For this review, take the finished solid that the model builds, in its own axes (mm). A direction names the side the tool comes from. Round coordinates to 2 decimals unless told otherwise and drop trailing zeros. Order: outer loops, then holes, each group sorted by start corner. A loop starts at its lowest first (then second) coordinate and runs counter-clockwise, first axis right, second up. Notation, with made-up numbers: (73.5, 36.5) - (85.5, 36.5) arc R21 ccw to (85.5, 74.5) - close; hole circle Ø4 at (-28.75, 1.5). An arc over 180 degrees is marked (long way). One line per item, written item: value.
```python
from build123d import *

# Parameters (mm, degrees)
BOSS_EXTRU_1_DEPTH = 20
ESQUISSE2_R        = 3
BOSS_EXTRU_2_DEPTH = 5


with BuildPart() as part:
    # Esquisse1 → Boss.-Extru.1 (new body)
    with BuildSketch(Plane(origin=(0, 0, 0), x_dir=(1, 0, 0), z_dir=(0, 1, 0))):
        Polygon((0, 0), (40, 0), (40, 2), (47, 2), (47, 7), (40, 7), (40, 28), (47, 28), (47, 31.5), (40, 31.5), (40, 37), (0, 37), (0, 31.5), (-7, 31.5), (-7, 28), (0, 28), align=None)
    extrude(amount=BOSS_EXTRU_1_DEPTH)

    # Esquisse2 → Boss.-Extru.2 (add)
    with BuildSketch(Plane(origin=(0, 0, -37), x_dir=(-1, 0, 0), z_dir=(0, 0, -1))):
        with Locations((-30, 10)):
            Circle(ESQUISSE2_R)
    extrude(amount=BOSS_EXTRU_2_DEPTH)


solid = part.part
```
Item 1: Wall thickness on line 1 (X direction, y = 7.25, z = -35); line 2 (Z direction, x = 25, y = 14); line 3 (Z direction, x = 44, y = 6.25): over which ranges is each line inside the solid? List them lowest first.
Returned:
line 1: 0 to 40
line 2: -37 to 0
line 3: -31.5 to -28, -7 to -2
Item 2: For P1, Ø2, axis at x = 45, y = 13.5, coming from the -Z side; P2, Ø0.6, axis at y = 13.5, z = -1.5, coming from the +X side; P3, Ø5.5, axis at x = 45, y = 9.5, coming from the +Z side; P4, Ø5, axis at x = 26.5, y = 14, coming from the +Z side, all flat-tipped, find the tip position at first contact; note any pin that passes through.
Returned:
P1: z = -31.5
P2: x = 40
P3: z = -2
P4: z = 0
Item 3: Take a section at B-B (y = 14). Write out the cut boundary in (x, z).
Returned:
outline: (-7, -31.5) - (0, -31.5) - (0, -37) - (40, -37) - (40, -31.5) - (47, -31.5) - (47, -28) - (40, -28) - (40, -7) - (47, -7) - (47, -2) - (40, -2) - (40, 0) - (0, 0) - (0, -28) - (-7, -28) - close
Item 4: Machinability: for faces 1 (the cylindrical face through (33, 10, -39)), 2 (the flat face through (-4, 10, -28)), 3 (the flat face through (40, 10, -34)), which of the approach directions +Z, -Z, +X, -X, +Y, -Y give a long, thin tool a straight path to every point of the face, cutting with its end or side? Answer none if there is none.
Returned:
face 1: -Z
face 2: +Z, -X, +Y, -Y
face 3: -Z, +X, +Y, -Y
Item 5: Take a section at A-A (x = 44.5). Write out the cut boundary in (y, z).
Returned:
outline: (0, -31.5) - (20, -31.5) - (20, -28) - (0, -28) - close; (0, -7) - (20, -7) - (20, -2) - (0, -2) - close
Item 6: Take a section at C-C (x = 30). Write out the cut boundary in (y, z).
Returned:
outline: (0, -37) - (7, -37) - (7, -42) - (13, -42) - (13, -37) - (20, -37) - (20, 0) - (0, 0) - close
Item 7: The part is to be moulded in two halves that separate along Z. For faces 4 (the flat face through (-3, 10, -31.5)), 5 (the flat face through (43, 10, -28)), 6 (the flat face through (20, 10, 0)), say which applies: +Z half, -Z half, draft (parallel to the pull), parting line (faces both ways), or undercut.
Returned:
face 4: -Z half
face 5: undercut
face 6: +Z half
Item 8: Take a section at D-D (z = -26). Write out the cut boundary in (x, y).
Returned:
outline: (0, 0) - (40, 0) - (40, 20) - (0, 20) - close
